Geometry check sheet. Reference: the model listing, model coordinates, mm. Face numbers are marked on the shaded views. A direction names the side the tool comes from. Coordinates: 2 decimals unless noted, no trailing zeros. Loops run counter-clockwise (first coordinate to the right, second up) from the corner with the lowest first, then second, coordinate; pieces in that order, holes last. Notation, with made-up numbers: (19, 53.25) - (72, 53.25) arc R33 cw to (72, 82.25) - close; hole circle Ø5 at (4.5, -5.5). An arc over 180 degrees is marked (long way). Write each question's results on one line, items separated by ' | '. Start each with the question number.
(1) Sectioned sample at D-D (x = -0.75). Enter the section's corners in (y, z).
(2) Access from +Z, -Z, +X, -X, +Y, -Y to the whole of each face (thin tool, end or side, straight path). Record for the marked faces 1, 2 and 3.
(3) Material ranges on probe 1 along X at (y, z) = (7, -1.15); probe 2 along Y at (x, z) = (-5, -1.35); probe 3 along Y at (x, z) = (-4.5, -0.55), recorded low to high.
(4) Sectioned sample at C-C (x = -5). Enter the section's corners in (y, z).
(5) Mould release check, pull along Y, two halves, no side actions. Record for the marked faces 4, 5 and 6: pulls with the +Y half, pulls with the -Y half, needs draft (parallel to the pull), parting line crosses it, or undercut.
(6) Go/stop test with flat-tipped pins: pin 1 Ø1 at (y, z) = (1, -2) entering from +X; pin 2 Ø1 at (y, z) = (0.5, -1.5) entering from -X; pin 3 Ø0.7 at (x, z) = (-7, -2) entering from -Y. Record where each tip stops, or that it passes through.
(7) Sectioned sample at A-A (y = 6). Enter the section's corners in (x, z).
(8) Sectioned sample at B-B (z = -1.75). Enter the section's corners in (x, y), plus the area to 3 significant figures.
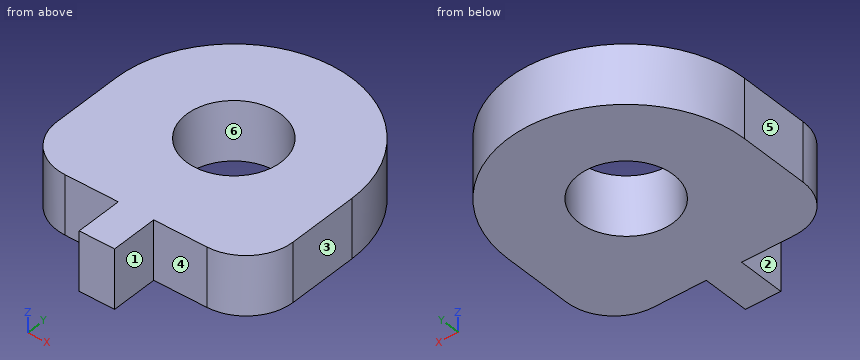
Autodesk Inventor part; units mm, degrees
ref_plane "YZ Plane" through (0, 0, 0) normal (1, 0, 0) x (0, 1, 0)
ref_plane "XZ Plane" through (0, 0, 0) normal (0, 1, 0) x (-1, 0, 0)
ref_plane "XY Plane" through (0, 0, 0) normal (0, 0, 1) x (1, 0, 0)
sketch "Sketch1" plane through (0, 0, 0) normal (0, 1, 0) x (-1, 0, 0)
  line L0 (0, 0) -> (0, -2.5)
  line L1 (0, -2.5) -> (10, -2.5)
  line L2 (10, -2.5) -> (10, 0)
  line L3 (10, 0) -> (0, 0)
  dimension "d0" = 2.5
  dimension "d1" = 10
  dimension "d2" = 90
  dimension "d3" = 2.5
extrude "Extrusion1" add sketch "Sketch1" along normal blind 12
sketch "Sketch4" plane through (0, 0, -2.5) normal (0, 0, -1) x (-1, 0, 0)
  line L0 (0, 0) -> (0, 2)
  line L1 (0, 0) -> (0, 12)
  line L2 (0, 2) -> (4, 2)
  line L3 (10, 0) -> (10, 12)
  line L4 (4, 2) -> (0, 0)
  line L5 (0, 0) -> (10, 0)
  line L6 (10, 0) -> (10, 2)
  line L7 (10, 2) -> (6, 2)
  line L8 (6, 2) -> (10, 0)
  dimension "d9" = 2
  dimension "d10" = 4
  dimension "d11" = 2
  dimension "d12" = 4
extrude "Extrusion3" cut sketch "Sketch4" against normal up to surface (2.5 mm away)
sketch "Sketch5" plane through (0, 12, -2.5) normal (0, 0, -1) x (-1, 0, 0)
  point P0 (0, -12)
sketch "Sketch6" plane through (0, 12, -2.5) normal (0, 0, -1) x (-1, 0, 0)
  line L0 (0, -10) -> (0, 0)
  line L1 (0, -5) -> (10, -5)
  line L2 (10, -10) -> (10, 0)
  line L3 (0, 0) -> (10, 0)
  line L4 (5, 0) -> (5, -10)
  circle A0 centre (5, -5) radius 2
  point P0 (0, -12)
  dimension "d15" = 4
extrude "Extrusion4" cut sketch "Sketch6" against normal up to surface (2.5 mm away) contours A0 L4 L1 | L1 L4 A0 | L4 A0 L1 | L1 A0 L4
fillet "Fillet1" radius 2 4 edges at (0, 12, -1.25) (0, 2, -1.25) (-10, 12, -1.25) (-10, 2, -1.25)
fillet "Fillet2" radius 0.5 1 edges at (0, 0, -1.25)
fillet "Fillet3" radius 0.5 1 edges at (-10, 0, -1.25)
sketch "Sketch7" plane through (-8, 12, 0) normal (0, 0, 1) x (1, 0, 0)
  circle A0 centre (3, -5) radius 2
  arc A1 (8, -2) -> (6, 0) centre (6, -2) ccw
  circle A2 centre (3, -5) radius 5
  line L0 (6, 0) -> (0, 0)
  arc A3 (-0.1056, -11.0528) -> (0.118, -12) centre (0.118, -11.5) ccw
  line L1 (0.118, -12) -> (5.882, -12)
  arc A4 (5.882, -12) -> (6.1056, -11.0528) centre (5.882, -11.5) ccw
  line L2 (6.1056, -11.0528) -> (4, -10)
  line L3 (4, -10) -> (6, -10)
  arc A5 (6, -10) -> (8, -8) centre (6, -8) ccw
  line L4 (8, -8) -> (8, -2)
  arc A6 (8, -2) -> (6, 0) centre (6, -2) ccw
  line L5 (0, 0) -> (6, 0)
  arc A7 (0, 0) -> (-2, -2) centre (0, -2) ccw
  line L6 (-2, -8) -> (-2, -2)
  arc A8 (-2, -8) -> (0, -10) centre (0, -8) ccw
  line L7 (0, -10) -> (2, -10)
  line L8 (2, -10) -> (-0.1056, -11.0528)
  circle A9 centre (3, -5) radius 2
  point P0 (8, -12)
  point P1 (-2, -5)
  point P2 (3, 0)
  point P3 (8, -5)
  point P4 (8, -2)
extrude "Extrusion5" cut sketch "Sketch7" against normal up to surface (2.5 mm away) contours L4 A2 L0 A1 | A2 L6 A7 L0
sketch "Sketch8" plane through (-8, 2, 0) normal (0, 0, 1) x (1, 0, 0)
  circle A0 centre (3, 5) radius 2
  arc A1 (8, 5) -> (-2, 5) centre (3, 5) ccw
  line L0 (-2, 2) -> (-2, 5)
  arc A2 (-2, 2) -> (0, 0) centre (0, 2) ccw
  line L1 (0, 0) -> (2, 0)
  line L2 (2, 0) -> (-0.1056, -1.0528)
  arc A3 (-0.1056, -1.0528) -> (0.118, -2) centre (0.118, -1.5) ccw
  line L3 (0.118, -2) -> (5.882, -2)
  arc A4 (5.882, -2) -> (6.1056, -1.0528) centre (5.882, -1.5) ccw
  line L4 (6.1056, -1.0528) -> (4, 0)
  line L5 (4, 0) -> (6, 0)
  arc A5 (6, 0) -> (8, 2) centre (6, 2) ccw
  line L6 (8, 2) -> (8, 5)
  line L7 (2, 0) -> (0, 0)
  line L8 (2, 0) -> (2, -2)
  line L9 (5.882, -2) -> (0.118, -2)
  line L10 (4, 0) -> (4, -2)
  line L11 (3, 0) -> (2.25, 0)
  line L12 (3, 0) -> (3.75, 0)
  line L13 (3.75, 0) -> (3.75, -2)
  line L14 (2.25, 0) -> (2.25, -2)
  line L15 (2.25, -2) -> (3.75, -2)
  line L16 (-0.1056, -1.0528) -> (2, 0)
  line L17 (2, 0) -> (4, 0)
  line L18 (2, -2) -> (4, -2)
  point P0 (8, -2)
  point P1 (2, -2)
  point P2 (2.25, 0)
  point P3 (2.25, -2)
  point P4 (3.75, 0)
  dimension "d25" = 0.75
  dimension "d26" = 0.75
extrude "Extrusion6" cut sketch "Sketch8" against normal up to surface (2.5 mm away) contours L4 A4 L3 L10 | L10 L3 L13 L17 | L8 L3 A3 L2 | L17 L14 L3 L8
properties part number "Knuckle Attachment DirectInsert"
Outcome:
1) outline: (2.44, -2.5) - (9.63, -2.5) - (9.63, 0) - (2.44, 0) - close
2) face 1: +Z, -Z, +X, -Y | face 2: +Z, -Z, -X, -Y | face 3: +Z, -Z, +X, +Y, -Y
3) probe 1: x = -10 to -7, -3 to 0 | probe 2: y = 0 to 5, 9 to 12 | probe 3: y = 0 to 5.06, 8.94 to 11.97
4) outline: (0, -2.5) - (5, -2.5) - (5, 0) - (0, 0) - close; (9, -2.5) - (12, -2.5) - (12, 0) - (9, 0) - close
5) face 4: pulls with the -Y half | face 5: needs draft | face 6: undercut
6) pin 1: stops at x = -4.25 | pin 2: stops at x = -5.75 | pin 3: stops at y = 2
7) outline: (-10, -2.5) - (-6.73, -2.5) - (-6.73, 0) - (-10, 0) - close; (-3.27, -2.5) - (0, -2.5) - (0, 0) - (-3.27, 0) - close
8) outline: (-10, 4) arc R2 ccw to (-8, 2) - (-5.75, 2) - (-5.75, 0) - (-4.25, 0) - (-4.25, 2) - (-2, 2) arc R2 ccw to (0, 4) - (0, 7) arc R5 ccw to (-10, 7) - close; hole circle Ø4 at (-5, 7) | area: 78.0 mm2
